Input: part model. Units: mm. Frame: model coordinates. Give positions to 0.01 mm unless a question says otherwise; leave off trailing zeros. Loops run counter-clockwise (first coordinate to the right, second up) from the corner with the lowest first, then second, coordinate; pieces in that order, holes last. Notation, with made-up numbers: M 44,81.25 L 73,81.25 A19 cw 73,102.25 Z; hole C 43,46 d11. An arc over 180 degrees is marked long. Answer as a JSON object with one key per item and string values. Group by question number.
1) Section query C-C on y = 1. Return loops of the section in (x, z).
2) Ray query, L1, parallel to Z at x = 43.5, y = 0.85; L2, parallel to X at y = 4.2, z = -26; L3, parallel to X at y = 2.05, z = -36. Return the intervals inside material, ascending.
3) Section query A-A on x = 40. Return loops of the section in (y, z).
4) Section query B-B on z = -43. Return loops of the section in (x, y).
5) Draft query along Z for faces 1 (the flat face through (69, 3, -76.708)), 2 (the cylindrical face through (127.275, 2.576, -25.133)), 3 (the cylindrical face through (124.3, 2.58, -2.87)), 4 (the flat face through (69, 5.08, -38)). Return one class per face: +Z half, -Z half, draft (parallel to the pull), parting line (faces both ways), or undercut.
6) Section query D-D on x = 107.5. Return loops of the section in (y, z).
7) First-contact query: P1, Ø1.5, axis at y = 4.5, z = -26.5, coming from the +X side; P2, Ø4, axis at x = 125.09, z = -24.45, coming from the +Y side; P3, Ø1.5, axis at y = 2, z = -35, coming from the +X side. Flat tips, straight axial feed; report the tip coordinate or a pass-through.
Autodesk Inventor part; units mm, degrees
ref_plane "YZ Plane" through (0, 0, 0) normal (1, 0, 0) x (0, 1, 0)
ref_plane "XZ Plane" through (0, 0, 0) normal (0, 1, 0) x (-1, 0, 0)
ref_plane "XY Plane" through (0, 0, 0) normal (0, 0, 1) x (1, 0, 0)
sketch "Sketch1" plane through (0, 0, 0) normal (0, 1, 0) x (-1, 0, 0)
  line L0 (0, 0) -> (-136.144, 0)
  line L1 (-136.144, 0) -> (-136.144, -76.708)
  line L2 (-136.144, -76.708) -> (0, -76.708)
  line L3 (0, -76.708) -> (0, 0)
  line L4 (-23.9341, -47.3101) -> (-44.2537, -47.1769)
  line L5 (-44.2537, -47.1769) -> (-44.1372, -29.3973)
  line L6 (-44.1372, -29.3973) -> (-23.8176, -29.5304)
  line L7 (-23.8176, -29.5304) -> (-23.9341, -47.3101)
  line L8 (-94.2086, -30.7353) -> (-94.2453, -45.9753)
  line L9 (-94.2453, -45.9753) -> (-111.5172, -45.9338)
  line L10 (-111.5172, -45.9338) -> (-111.4806, -30.6938)
  line L11 (-111.4806, -30.6938) -> (-94.2086, -30.7353)
  line L12 (-68.072, -76.708) -> (-68.072, 0)
  line L13 (-136.144, -76.708) -> (-68.072, -76.708)
  line L14 (-102.108, -76.708) -> (-103.5543, 0)
  line L15 (-111.4806, -30.6938) -> (-94.2453, -45.9753)
  line L16 (-94.2086, -30.7353) -> (-111.5172, -45.9338)
  line L17 (-44.1372, -29.3973) -> (-23.9341, -47.3101)
  line L18 (-44.2537, -47.1769) -> (-23.8176, -29.5304)
  line L19 (-68.072, -76.708) -> (0, -76.708)
  line L20 (-34.036, -76.708) -> (-34.036, 0)
  line L21 (-68.072, -38.354) -> (0, -38.354)
  line L22 (-68.072, -38.354) -> (-136.144, -38.354)
  dimension "d0" = 136.144
  dimension "d1" = 76.708
  dimension "d2" = 20.32
  dimension "d3" = 17.78
  dimension "d4" = 15.24
  dimension "d6" = 17.272
extrude "Extrusion1" add sketch "Sketch1" along normal blind 5.08 contours L3 L21 L7 L6 L20 L0 | L20 L6 L5 L21 L12 L0 | L3 L2 L20 L4 L7 L21 | L12 L22 L8 L11 L14 L0 | L14 L11 L10 L22 L1 L0 | L21 L5 L4 L20 L2 L12 | L12 L2 L14 L9 L8 L22 | L22 L10 L9 L14 L2 L1
sketch "Sketch2" plane through (0, 5.08, 0) normal (0, 1, 0) x (1, 0, 0)
  line L0 (0, 76.708) -> (0, 0)
  line L1 (0, 0) -> (136.144, 0)
  line L2 (136.144, 0) -> (136.144, 76.708)
  circle A0 centre (128.5715, 55.9707) radius 2.286
  circle A1 centre (125.0945, 24.4461) radius 2.286
  circle A2 centre (8.0361, 53.8336) radius 2.286
  circle A3 centre (12.3665, 25.1981) radius 2.286
  line L3 (127.3823, 10.0745) -> (136.144, 10.0745)
  line L4 (127.3823, 10.0745) -> (0, 10.0745)
  line L5 (0, 76.708) -> (8.0361, 10.0745)
  line L6 (136.144, 76.708) -> (127.3823, 10.0745)
  line L7 (8.0361, 10.0745) -> (8.0361, 10.16)
  line L8 (18.1961, 0) -> (117.2223, 0)
  arc A4 (8.0361, 10.16) -> (18.1961, 0) centre (18.1961, 10.16) ccw
  line L9 (127.3823, 10.0745) -> (127.3823, 10.16)
  arc A5 (117.2223, 0) -> (127.3823, 10.16) centre (117.2223, 10.16) ccw
  line L10 (0, 76.708) -> (0, 0)
  line L11 (0, 0) -> (136.144, 0)
  line L12 (136.144, 0) -> (136.144, 76.708)
  line L13 (136.144, 76.708) -> (0, 76.708)
  line L14 (23.9341, 47.3101) -> (44.2537, 47.1769)
  line L15 (44.2537, 47.1769) -> (44.1372, 29.3973)
  line L16 (44.1372, 29.3973) -> (23.8176, 29.5304)
  line L17 (23.8176, 29.5304) -> (23.9341, 47.3101)
  line L18 (94.2453, 45.9753) -> (111.5172, 45.9338)
  line L19 (111.5172, 45.9338) -> (111.4806, 30.6938)
  line L20 (111.4806, 30.6938) -> (94.2086, 30.7353)
  line L21 (94.2086, 30.7353) -> (94.2453, 45.9753)
  line L22 (125.0945, 24.4461) -> (12.3665, 25.1981)
  point P0 (8.0361, 0)
  point P1 (8.0365, 10.0745)
  point P2 (127.382, 10.0745)
  point P3 (117.2223, 0)
  dimension "d9" = 10.16
  dimension "d10" = 10.16
  dimension "d11" = 4.572
  dimension "d12" = 4.572
extrude "Extrusion2" cut sketch "Sketch2" against normal blind 5.08 contours L5 L4 L0 | L4 A4 L1 L0 | L2 L3 L6 | L3 L2 L1 A5 | A0 | A1 | A3 | A2
properties part number "chair power plate"
Output:
{
 "1": {"outline": "M 0,-76.71 L 136.14,-76.71 L 127.38,-10.07 A10.16 ccw 117.22,0 L 18.2,0 A10.16 ccw 8.04,-10.07 Z; hole C 8.04,-53.83 d4.57; hole C 12.37,-25.2 d4.57; hole M 23.82,-29.53 L 23.93,-47.31 L 44.25,-47.18 L 44.14,-29.4 Z; hole M 94.21,-30.74 L 94.25,-45.98 L 111.52,-45.93 L 111.48,-30.69 Z; hole C 125.09,-24.45 d4.57; hole C 128.57,-55.97 d4.57"},
 "2": {"L1": "z = -76.71 to -47.18, -29.4 to 0", "L2": "x = 6.12 to 10.23, 14.51 to 123.42, 126.77 to 129.48", "L3": "x = 4.91 to 23.86, 44.18 to 94.22, 111.49 to 130.79"},
 "3": {"outline": "M 0,-76.71 L 5.08,-76.71 L 5.08,-47.2 L 0,-47.2 Z; M 0,-29.42 L 5.08,-29.42 L 5.08,0 L 0,0 Z"},
 "4": {"outline": "M 4.07,0 L 23.91,0 L 23.91,5.08 L 4.07,5.08 Z; M 44.23,0 L 94.24,0 L 94.24,5.08 L 44.23,5.08 Z; M 111.51,0 L 131.71,0 L 131.71,5.08 L 111.51,5.08 Z"},
 "5": {"face 1": "-Z half", "face 2": "undercut", "face 3": "+Z half", "face 4": "draft"},
 "6": {"outline": "M 0,-76.71 L 5.08,-76.71 L 5.08,-45.94 L 0,-45.94 Z; M 0,-30.7 L 5.08,-30.7 L 5.08,0 L 0,0 Z"},
 "7": {"P1": "stops at x = 129.64", "P2": "passes through", "P3": "stops at x = 130.76"}
}
